Build history of the part. All positions in model axes, mm. Face numbers are marked on the shaded views. Round coordinates to 2 decimals unless told otherwise and drop trailing zeros. Loops run counter-clockwise (first coordinate to the right, second up) from the corner with the lowest first, then second, coordinate; pieces in that order, holes last.
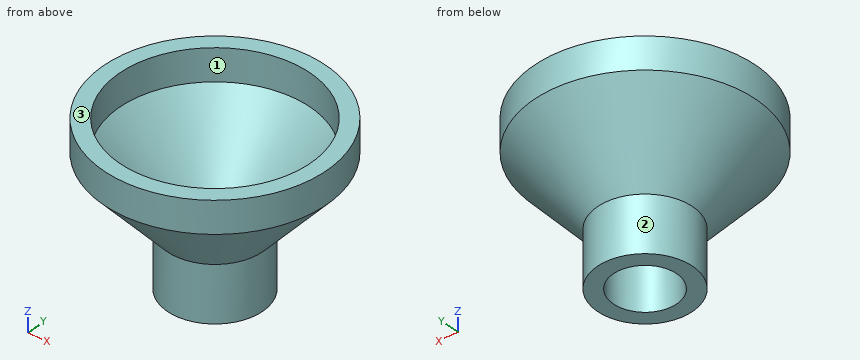
from build123d import *

# Parameters (mm, degrees)
F0_W     = 3.175
F0_H     = 6.35
F0_H_2   = 11.083638
F2_R     = 9.040902
F3_DEPTH = 9.525
F4_R     = 9.539088
F5_DEPTH = 25.4


with BuildPart() as f1:
    # F0 (on Right) → F1 (revolve)
    with BuildSketch(Plane.YZ):
        with Locations((20.6375, 3.175)):
            Rectangle(F0_W, F0_H)
        Polygon((9.525, -14.316362), (22.225, 0), (19.05, 0), (6.35, -14.316362), align=None)
        with Locations((7.9375, -19.858181)):
            Rectangle(F0_W, F0_H_2)
    revolve(axis=Axis((0, 0, -21.81005), (0, 0, 1)))


with BuildPart() as f3:
    # F2 (on Top) → F3 (new body)
    with BuildSketch(Plane.XY):
        Circle(F2_R)
    extrude(amount=F3_DEPTH)

    # F4 (on Top) → F5 (join)
    with BuildSketch(Plane.XY):
        Circle(F4_R)
    extrude(amount=F5_DEPTH)


solid = f1.part
(1) Pin check, flat tips, straight feed: P1, Ø3, axis at x = 12.5, z = 2, coming from the -Y side; P2, Ø6, axis at x = -5.5, z = 2, coming from the +Y side; P3, Ø11.5, axis at x = 0, y = 0, coming from the +Z side; P4, Ø5, axis at x = -16.5, y = -16.5, coming from the -Z side. Stop position of each tip, or through.
Responses:
P1: stops at y = -19.31
P2: stops at y = 22.08
P3: passes through
P4: stops at z = -1.57
(2) Slice it at C-C on z = -22.5. List the corners of the cut face in (x, y) (3 decimals), plus the area to 3 significant figures.
Responses:
outline: circle Ø19.05 at (0, 0); hole circle Ø12.7 at (0, 0)
area: 158 mm2
(3) Slice it at D-D on z = 3.5. List the corners of the cut face in (x, y) (3 decimals), plus the area to 3 significant figures.
Responses:
outline: circle Ø44.45 at (0, 0); hole circle Ø38.1 at (0, 0)
area: 412 mm2
(4) Pull direction Y, two halves, no side cores. Call the marked faces 1, 2 and 3: +Y half, -Y half, draft (parallel to the pull), parting line (faces both ways), or undercut.
Responses:
face 1: undercut
face 2: parting line
face 3: draft
(5) Slice it at A-A on y = 0. List the corners of the cut face in (x, z) (3 decimals).
Responses:
outline: (-22.225, 0) - (-9.525, -14.316) - (-9.525, -25.4) - (-6.35, -25.4) - (-6.35, -14.316) - (-19.05, 0) - (-19.05, 6.35) - (-22.225, 6.35) - close; (6.35, -25.4) - (9.525, -25.4) - (9.525, -14.316) - (22.225, 0) - (22.225, 6.35) - (19.05, 6.35) - (19.05, 0) - (6.35, -14.316) - close
(6) Probe line 1 (X direction, y = 0, z = 5) (3 decimals); line 2 (Y direction, x = 0, z = -19) (3 decimals). List the from-to ranges inside material, lowest first.
Responses:
line 1: x = -22.225 to -19.05, 19.05 to 22.225
line 2: y = -9.525 to -6.35, 6.35 to 9.525
